```python
from build123d import *

# Parameters (mm, degrees)
BOSS_EXTRUDE1_DEPTH = 10.9
CHAMFER1_SIZE       = 1
SKETCH2_R           = 39.716531346
CUT_EXTRUDE1_DEPTH  = 0.65


with BuildPart() as part:
    # Sketch1 → Boss-Extrude1 (new body)
    with BuildSketch(Plane(origin=(0, 0, 0), x_dir=(1, 0, 0), z_dir=(0, 1, 0))):
        with BuildLine():
            ThreePointArc((-3.336791258, -24.776315789), (0, -25), (3.336791258, -24.776315789))
            ThreePointArc((3.336791258, -24.776315789), (4.47137835, -26.262417453), (4.980726164, -28.061403509))
            ThreePointArc((4.980726164, -28.061403509), (0, -28.5), (-4.980726164, -28.061403509))
            ThreePointArc((-4.980726164, -28.061403509), (-4.47137835, -26.262417453), (-3.336791258, -24.776315789))
        make_face()
    extrude(amount=BOSS_EXTRUDE1_DEPTH)

    # Chamfer1
    chamfer1_edges = [part.edges().sort_by_distance(p)[0] for p in [
        (0, 10.9, 28.5),
    ]]
    chamfer(chamfer1_edges, length=CHAMFER1_SIZE)

    # Sketch2 → Cut-Extrude1 (cut)
    with BuildSketch(Plane(origin=(0, 10.9, 0), x_dir=(1, 0, 0), z_dir=(0, 1, 0))):
        Circle(SKETCH2_R)
    extrude(amount=-CUT_EXTRUDE1_DEPTH, mode=Mode.SUBTRACT)


solid = part.part
```
The listing builds one solid part. Answer for the finished solid, in the listing's coordinates (mm). Coordinates: 2 decimals unless noted, no trailing zeros. Write each loop counter-clockwise with the first axis right and the second up, starting at its lowest first coordinate (ties: lowest second). Pieces come first, ordered by that corner, then holes. Notation, with made-up numbers: (85.25, 0.5) - (135.25, 0.5) arc R14 cw to (135.25, 12.5) - close; hole circle Ø8 at (89.5, 70). An arc over 180 degrees is marked (long way). One line per item, written item: value.
1) Find section B-B (z = 26.1). Give the vertices of the cut face in (x, y), and give its area (3 significant figures).
Geometry check:
outline: (-4.39, 0) - (4.39, 0) - (4.39, 10.25) - (-4.39, 10.25) - close
area: 89.9 mm2
2) Consider line 1 along X through (y, z) = (2.75, 26.25); line 2 along Z through (x, y) = (3.5, 9); line 3 along X through (y, z) = (8.5, 26.6). Determine where each line is inside the solid, lowest interval first. Write a range as from..to.
Geometry check:
line 1: x = -4.47..4.47
line 2: z = 24.93..28.28
line 3: x = -4.62..4.62
3) For a pull along X with two mould halves and no side action, classify faces 1 (the cylindrical face through (-4.483, 5.053, 26.286)), 2 (the cylindrical face through (4.46, 5.05, 26.24)), 3 (the cylindrical face through (0, 5, 25)) as pulls with the +X half, pulls with the -X half, needs draft (parallel to the pull), parting line crosses it, or undercut.
Geometry check:
face 1: pulls with the -X half
face 2: pulls with the +X half
face 3: undercut
4) Find section A-A (y = 8). Give the vertices of the cut face in (x, z).
Geometry check:
outline: (-4.98, 28.06) arc R5 ccw to (-3.34, 24.78) arc R25 cw to (3.34, 24.78) arc R5 ccw to (4.98, 28.06) arc R28.5 ccw to start
